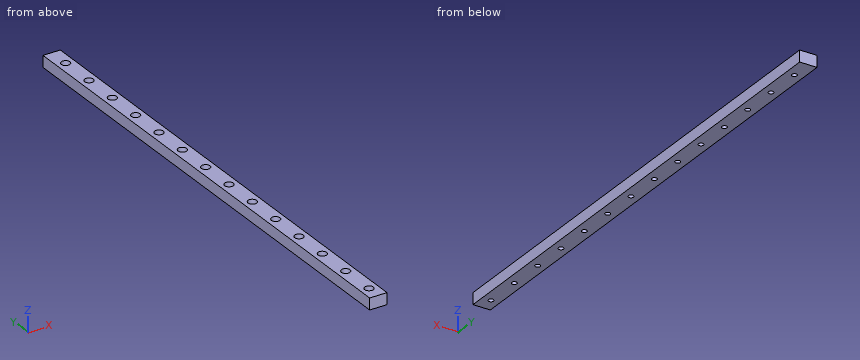
```python
from build123d import *

# Parameters (mm, degrees)
SKETCH_1_W             = 12
SKETCH_1_H             = 8
EXTRUDE_1_DEPTH        = 350
SKETCH_2_R             = 3
CUT_EXTRUDE_1_DEPTH    = 4.5
SKETCH_3_R             = 1.75
CUT_EXTRUDE_2_DEPTH    = 4.5
PATTERN_LINEAR_1_COUNT = 14
PATTERN_LINEAR_1_PITCH = 25


with BuildPart() as part:
    # 草图1 → 凸台-拉伸1 (new body)
    with BuildSketch(Plane(origin=(0, 0, 0), x_dir=(1, 0, 0), z_dir=(0, 1, 0))):
        Rectangle(SKETCH_1_W, SKETCH_1_H)
    extrude(amount=EXTRUDE_1_DEPTH)

    # 草图2 → 切除-拉伸1 (cut)
    with BuildSketch(Plane.XY.offset(4)):
        with Locations((0, 10)):
            Circle(SKETCH_2_R)
    cut_extrude_1 = extrude(amount=-CUT_EXTRUDE_1_DEPTH, mode=Mode.SUBTRACT)

    # 草图3 → 切除-拉伸2 (cut)
    with BuildSketch(Plane.XY.offset(-0.5)):
        with Locations((0, 10)):
            Circle(SKETCH_3_R)
    cut_extrude_2 = extrude(amount=-CUT_EXTRUDE_2_DEPTH, mode=Mode.SUBTRACT)

    # 阵列(线性)1: 切除-拉伸1, 切除-拉伸2 ×14
    with Locations(*[(0, i * PATTERN_LINEAR_1_PITCH, 0) for i in range(1, PATTERN_LINEAR_1_COUNT)]):
        add(cut_extrude_1, mode=Mode.SUBTRACT)
        add(cut_extrude_2, mode=Mode.SUBTRACT)


solid = part.part
```
Part model, mm, in its own coordinate system. Coordinates: 2 decimals unless noted, no trailing zeros.
Item 1: Slice it at A-A (z = 0.75). Count the separate pieces of the cut face and the enclosed holes in it, and give its area (3 significant figures).
Item 2: Probe line 1 (X direction, y = 110, z = 1.35); line 2 (X direction, y = 235, z = -2.9). List the from-to ranges inside material, lowest first.
Item 3: Pin check, flat tips, straight feed: pin 1 (3 mm diameter, centred on x = -0.5, y = 86, fed in from +Z); pin 2 (4.5 mm diameter, centred on x = 0, y = 35, fed in from -Z); pin 3 (2 mm diameter, centred on x = 0, y = 110, fed in from +Z). Stop position of each tip, or through.
Results found:
1. separate pieces: 1
1. enclosed holes: 14
1. area: 3,800 mm2
2. line 1: x = -6 to -3, 3 to 6
2. line 2: x = -6 to -1.75, 1.75 to 6
3. pin 1: stops at z = -0.5
3. pin 2: stops at z = -4
3. pin 3: passes through
